```python
from build123d import *

# Parameters (mm, degrees)
F1_DEPTH = 25.4
F3_DEPTH = 35.814
F4_R     = 17.384083
F5_DEPTH = 4.572


with BuildPart() as f1:
    # F0 (on Top) → F1 (new body)
    with BuildSketch(Plane.XY):
        Polygon((-35.676657, -9.338491), (18.646077, 59.587132), (-68.206631, 72.169188), align=None)
    extrude(amount=F1_DEPTH)

    # F2 (on face) → F3 (join)
    with BuildSketch(Plane.XY.offset(25.4)):
        with BuildLine():
            Line((-51.654875, 30.696816), (-54.485089, 37.788251))
            ThreePointArc((-54.485089, 37.788251), (-53.363226, 34.125499), (-51.654875, 30.696816))
        make_face()
        with BuildLine():
            ThreePointArc((-54.485089, 37.788251), (-34.270187, 65.84384), (-8.542018, 42.739302))
            ThreePointArc((-8.542018, 42.739302), (-25.528601, 20.357725), (-51.654875, 30.696816))
            Line((-51.654875, 30.696816), (-35.676657, -9.338491))
            Line((-35.676657, -9.338491), (18.646077, 59.587132))
            Line((18.646077, 59.587132), (-68.206631, 72.169188))
            Line((-68.206631, 72.169188), (-54.485089, 37.788251))
        make_face()
        with BuildLine():
            ThreePointArc((-51.654875, 30.696816), (-25.528601, 20.357725), (-8.542018, 42.739302))
            ThreePointArc((-8.542018, 42.739302), (-34.270187, 65.84384), (-54.485089, 37.788251))
            Line((-54.485089, 37.788251), (-51.654875, 30.696816))
        make_face()
    extrude(amount=F3_DEPTH)

    # F4 (on face) → F5 (join)
    with BuildSketch(Plane.XY.offset(61.214)):
        with Locations((-37.021548, 43.473128)):
            Circle(F4_R)
    extrude(amount=F5_DEPTH)


solid = f1.part
```
Could you check a few things on this model? Use its own coordinates, in mm. A direction names the side the tool comes from. Round coordinates to 2 decimals unless told otherwise and drop trailing zeros. Loops run counter-clockwise (first coordinate to the right, second up) from the corner with the lowest first, then second, coordinate; pieces in that order, holes last. Notation, with made-up numbers: (45, -9) -> (97, -9) arc R31 ccw to (97, 21) -> close; hole circle Ø4 at (17, 0). An arc over 180 degrees is marked (long way). One line per question, with ' | ' between items.
(1) If I drill on probe 1 along Z at (x, y) = (-34, 15.5); probe 2 along Y at (x, z) = (-6, 12); probe 3 along Y at (x, z) = (-7, 36), over which ranges is the centre line in solid material (lowest first)?
Model answer:
probe 1: z = 0 to 61.21 | probe 2: y = 28.32 to 63.16 | probe 3: y = 27.05 to 63.3
(2) If we section it at C-C on y = 32: List the corners of the cut face in (x, z) for me, and give its area (3 significant figures).
Model answer:
outline: (-52.39, 25.4) -> (-52.17, 25.4) -> (-52.17, 0) -> (-3.1, 0) -> (-3.1, 61.21) -> (-23.96, 61.21) -> (-23.96, 65.79) -> (-50.08, 65.79) -> (-50.08, 61.21) -> (-52.39, 61.21) -> close | area: 3,130 mm^2
(3) For pin 1 Ø10 at (x, z) = (-18.5, 27.5) entering from +Y; pin 2 Ø1 at (x, y) = (-40.5, 8.5) entering from -Z; pin 3 Ø12 at (x, z) = (-1.5, 48) entering from -Y; pin 4 Ø5 at (y, z) = (46, 16) entering from -X, each with a flat end and sliding along its axis, tell me the tip position at first contact or that it passes through.
Model answer:
pin 1: stops at y = 65.69 | pin 2: stops at z = 0 | pin 3: stops at y = 26.41 | pin 4: stops at x = -58.76
(4) For faces 1 (the face through (-25, 41, 0)), 2 (the face through (-16, 41, 61.214)), which set-ups out of +Z, -Z, +X, -X, +Y, -Y let a thin tool reach every point of the face, with its end or its side?
Model answer:
face 1: -Z, +X, -X, +Y, -Y | face 2: +Z
(5) If we section it at B-B on z = 6.5: List the corners of the cut face in (x, y) for me.
Model answer:
outline: (-68.21, 72.17) -> (-35.68, -9.34) -> (18.65, 59.59) -> close
(6) If we section it at D-D on z = 47.5: List the corners of the cut face in (x, y) for me.
Model answer:
outline: (-68.21, 72.17) -> (-54.49, 37.79) arc R23.24 ccw to (-51.65, 30.7) -> (-35.68, -9.34) -> (18.65, 59.59) -> close
(7) If we section it at A-A on x = -43.5: List the corners of the cut face in (y, z) for me, and give its area (3 significant figures).
Model answer:
outline: (10.26, 0) -> (68.59, 0) -> (68.59, 61.21) -> (59.6, 61.21) -> (59.6, 65.79) -> (27.34, 65.79) -> (27.34, 61.21) -> (10.26, 61.21) -> close | area: 3,720 mm^2
